from build123d import *

# Parameters (mm, degrees)
BOSS_EXTRUDE2_DEPTH = 5.08
FILLET3_R           = 2.54
FILLET4_R           = 2.54


with BuildPart() as part:
    # Sketch3 → Boss-Extrude2 (new body)
    with BuildSketch(Plane.XY):
        with BuildLine():
            Line((0.14834484, -16.543006694), (-0.005888561, -3.843943262))
            add(Edge.make_bspline(
                [(6.500180425, 78.706993306), (18.901808207, 35.989935529), (-0.005888561, -3.843943262)],
                knots=[0, 0, 0, 1, 1, 1], degree=2))
            Line((6.500180425, 78.706993306), (6.500180425, 85.056993306))
            Line((6.500180425, 85.056993306), (18.406430425, 85.056993306))
            Line((18.406430425, 85.056993306), (22.903074533, 81.262968128))
            Line((22.903074533, 81.262968128), (27.983074533, 81.262968128))
            Line((27.983074533, 81.262968128), (32.479718641, 85.056993306))
            Line((32.479718641, 85.056993306), (44.385968641, 85.056993306))
            Line((44.385968641, 85.056993306), (44.385968641, 78.706993306))
            add(Edge.make_bspline(
                [(44.385968641, 78.706993306), (31.984340858, 35.989935529), (50.892037627, -3.843943262)],
                knots=[0, 0, 0, 1, 1, 1], degree=2))
            Line((50.892037627, -3.843943262), (50.737804225, -16.543006694))
            Line((50.737804225, -16.543006694), (48.197804225, -16.543006694))
            Line((48.197804225, -16.543006694), (48.197804225, -21.623006694))
            Line((48.197804225, -21.623006694), (43.117804225, -21.623006694))
            Line((43.117804225, -21.623006694), (43.117804225, -16.543006694))
            Line((43.117804225, -16.543006694), (40.577804225, -16.543006694))
            add(Edge.make_bspline(
                [(27.983074533, 5.062968128), (40.683819064, -1.22119794), (40.577804225, -16.543006694)],
                knots=[0, 0, 0, 1, 1, 1], degree=2))
            Line((27.983074533, 5.062968128), (27.983074533, 55.862968128))
            Line((27.983074533, 55.862968128), (22.903074533, 55.862968128))
            Line((22.903074533, 55.862968128), (22.903074533, 5.062968128))
            add(Edge.make_bspline(
                [(22.903074533, 5.062968128), (10.202330001, -1.22119794), (10.30834484, -16.543006694)],
                knots=[0, 0, 0, 1, 1, 1], degree=2))
            Line((10.30834484, -16.543006694), (7.76834484, -16.543006694))
            Line((7.76834484, -16.543006694), (7.76834484, -21.623006694))
            Line((7.76834484, -21.623006694), (2.68834484, -21.623006694))
            Line((2.68834484, -21.623006694), (2.68834484, -16.543006694))
            Line((2.68834484, -16.543006694), (0.14834484, -16.543006694))
        make_face()
    extrude(amount=BOSS_EXTRUDE2_DEPTH)

    # Fillet3
    fillet3_edges = [part.edges().sort_by_distance(p)[0] for p in [
        (6.500180425, 85.056993306, 2.54),
        (44.385968641, 85.056993306, 2.54),
    ]]
    fillet(fillet3_edges, radius=FILLET3_R)

    # Fillet4
    fillet4_edges = [part.edges().sort_by_distance(p)[0] for p in [
        (27.983074533, 5.062968128, 2.54),
        (22.903074533, 5.062968128, 2.54),
    ]]
    fillet(fillet4_edges, radius=FILLET4_R)


solid = part.part
Source: CAD feature listing. Evaluate the final solid. Frame: model axes, mm. A direction names the side the tool comes from. Round coordinates to 2 decimals unless told otherwise and drop trailing zeros. Loops run counter-clockwise (first coordinate to the right, second up) from the corner with the lowest first, then second, coordinate; pieces in that order, holes last. Notation, with made-up numbers: (-11, -10.75) - (47, -10.75) arc R17 ccw to (47, -4.75) - close; hole circle Ø10 at (-12.75, 21.5). An arc over 180 degrees is marked (long way). Write item = value, one per line. Start each with the question number.
Item 1: Material intervals for line 1 (X direction, y = 45, z = 4.15); line 2 (X direction, y = -17, z = 4.8); line 3 (Y direction, x = 24.5, z = 2.5), sorted ascending.
Item 2: Section query A-A on x = 24. Output: boundary loops of the cut face in (y, z).
Item 3: First-contact query: pin 1 Ø3 at (x, z) = (1, 1.5) entering from -Y; pin 2 Ø2.5 at (x, z) = (24, 2) entering from +Y; pin 3 Ø2.5 at (y, z) = (-18, 2.5) entering from -X. Flat tips, straight axial feed; report the tip coordinate or a pass-through.
Item 4: Reachability of faces 4 (the face through (1, -16.543, 3)), 5 (the face through (25, 55.863, 3)), 6 (the face through (30.2, 83.133, 2.504)) from +Z, -Z, +X, -X, +Y, -Y: full face, straight path, thin tool, end or side. Return the list, or none.
Item 5: Mould query, pull axis X, two halves, no side actions, for faces 1 (the face through (46, -21.623, 3)), 2 (the face through (44.386, 81, 3)), 3 (the face through (7.768, -19, 3)). Classes: released by +X, released by -X, zero draft, split by the parting line, or undercut.
Results list:
q1.line_1 = 11.41 to 22.9, 27.98 to 39.47
q1.line_2 = 2.69 to 7.77, 43.12 to 48.2
q1.line_3 = 55.86 to 81.26
q2.outline = (55.86, 0) - (81.26, 0) - (81.26, 5.08) - (55.86, 5.08) - close
q3.pin_1 = -16.54
q3.pin_2 = 81.39
q3.pin_3 = 2.69
q4.face_4 = +Z, -Z, -X, -Y
q4.face_5 = +Z, -Z, -Y
q4.face_6 = +Z, -Z, +Y
q5.face_1 = zero draft
q5.face_2 = released by +X
q5.face_3 = undercut
